```python
from build123d import *

# Parameters (mm, degrees)
ESBO_O1_R                = 7.65
RESSALTO_EXTRUS_O1_DEPTH = 24
ESBO_O2_R                = 1.75
CORTE_EXTRUS_O1_DEPTH    = 20


with BuildPart() as part:
    # Esboço1 → Ressalto-extrusão1 (new body)
    with BuildSketch(Plane.XY):
        with BuildLine():
            Line((-10.95445115, -1), (-20, -1))
            Line((-20, -1), (-20, -11))
            Line((-20, -11), (0, -11))
            Line((0, -11), (20, -11))
            Line((20, -11), (20, -1))
            Line((20, -1), (10.95445115, -1))
            ThreePointArc((10.95445115, -1), (0, 11), (-10.95445115, -1))
        make_face()
        Circle(ESBO_O1_R, mode=Mode.SUBTRACT)
    extrude(amount=RESSALTO_EXTRUS_O1_DEPTH)

    # Esboço2 → Corte-extrusão1 (cut)
    with BuildSketch(Plane.XZ.offset(11)):
        with Locations(Location((15, 19.5, 0), (0, 0, 270))):
            Circle(ESBO_O2_R)
        with Locations(Location((15, 4.5, 0), (0, 0, 270))):
            Circle(ESBO_O2_R)
        with Locations(Location((-15, 4.5, 0), (0, 0, 270))):
            Circle(ESBO_O2_R)
        with Locations(Location((-15, 19.5, 0), (0, 0, 270))):
            Circle(ESBO_O2_R)
    extrude(amount=-CORTE_EXTRUS_O1_DEPTH, mode=Mode.SUBTRACT)


solid = part.part
```
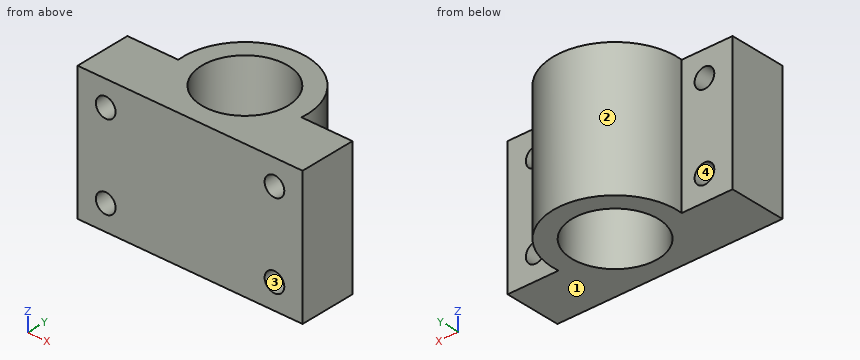
The listing builds one solid part. Answer for the finished solid, in the listing's coordinates (mm). Face numbers are marked on the shaded views. Round coordinates to 2 decimals unless told otherwise and drop trailing zeros. Order: outer loops, then holes, each group sorted by start corner. A loop starts at its lowest first (then second) coordinate and runs counter-clockwise, first axis right, second up. Notation, with made-up numbers: (72.25, 89) -> (93.25, 89) arc R34 cw to (93.25, 127) -> close; hole circle Ø10 at (89, 35.25). An arc over 180 degrees is marked (long way). Answer as CSV lines item,"result". Start each with the question number.
(1) Flat-ended cylindrical pins translate along their axes: pin 1 Ø10 at (x, z) = (17, 17) entering from +Y; pin 2 Ø12 at (x, z) = (15, 7.5) entering from +Y. Find the tip coordinate at first contact, or state that the pin passes through.
(2) The part is cut by section B-B (x = 0). Determine the outline of the cut face in (y, z), then the cut area to 3 significant figures.
(3) The part is cut by section D-D (x = -15). Determine the outline of the cut face in (y, z), then the cut area to 3 significant figures.
(4) For a pull along Z with two mould halves and no side action, classify the marked faces 1, 2, 3 and 4 as +Z half, -Z half, draft (parallel to the pull), parting line (faces both ways), or undercut.
(5) The part is cut by section A-A (z = 19.5). Determine the outline of the cut face in (x, y), then the cut area to 3 significant figures.
(6) The part is cut by section C-C (y = -3.75). Determine the outline of the cut face in (x, z), then the cut area to 3 significant figures.
(7) Find the intervals of material crossed by probe 1 along X at (y, z) = (-7.75, 19.5); probe 2 along X at (y, z) = (-5.5, 4.5); probe 3 along Z at (x, y) = (14, -1.75), in increasing order. Write a range as from..to.
Evaluation:
1,pin 1,"y = -1"
1,pin 2,"y = 6.32"
2,outline,"(-11, 0) -> (-7.65, 0) -> (-7.65, 24) -> (-11, 24) -> close; (7.65, 0) -> (11, 0) -> (11, 24) -> (7.65, 24) -> close"
2,area,"161 mm²"
3,outline,"(-11, 0) -> (-1, 0) -> (-1, 2.75) -> (-11, 2.75) -> close; (-11, 6.25) -> (-1, 6.25) -> (-1, 17.75) -> (-11, 17.75) -> close; (-11, 21.25) -> (-1, 21.25) -> (-1, 24) -> (-11, 24) -> close"
3,area,"170 mm²"
4,face 1,"-Z half"
4,face 2,"draft"
4,face 3,"undercut"
4,face 4,"undercut"
5,outline,"(-20, -11) -> (-16.75, -11) -> (-16.75, -1) -> (-20, -1) -> close; (-13.25, -11) -> (13.25, -11) -> (13.25, -1) -> (10.95, -1) arc R11 ccw (long way) to (-10.95, -1) -> (-13.25, -1) -> close; (16.75, -11) -> (20, -11) -> (20, -1) -> (16.75, -1) -> close; hole circle Ø15.3 at (0, 0)"
5,area,"358 mm²"
6,outline,"(-20, 0) -> (-6.67, 0) -> (-6.67, 24) -> (-20, 24) -> close; (6.67, 0) -> (20, 0) -> (20, 24) -> (6.67, 24) -> close; hole circle Ø3.5 at (-15, 4.5); hole circle Ø3.5 at (-15, 19.5); hole circle Ø3.5 at (15, 4.5); hole circle Ø3.5 at (15, 19.5)"
6,area,"601 mm²"
7,probe 1,"-20..-16.75, -13.25..13.25, 16.75..20"
7,probe 2,"-20..-16.75, -13.25..-5.32, 5.32..13.25, 16.75..20"
7,probe 3,"0..3.06, 5.94..18.06, 20.94..24"
